from build123d import *

# Parameters (mm, degrees)
BOSS_EXTRUDE4_DEPTH = 50
SKETCH7_R           = 1.75
CUT_EXTRUDE1_DEPTH  = 59.719147195
SKETCH8_R           = 0.75
SKETCH8_W           = 11.8
SKETCH8_H           = 22.5
BOSS_EXTRUDE5_DEPTH = 6
SKETCH9_R           = 4.05
BOSS_EXTRUDE6_DEPTH = 8
FILLET1_R           = 3


with BuildPart() as part:
    # Sketch6 → Boss-Extrude4 (new body)
    with BuildSketch(Plane.XZ):
        with BuildLine():
            Line((-1, 25.784833184), (-1, 12.785954208))
            ThreePointArc((-1, 12.785954208), (-12.825, 0), (-1, -12.785954208))
            Line((-1, -12.785954208), (-1, -25.784833184))
            Line((-1, -25.784833184), (-6, -25.784833184))
            Line((-6, -25.784833184), (-6, -16.784833184))
            ThreePointArc((-6, -16.784833184), (-17.825, 0), (-6, 16.784833184))
            Line((-6, 16.784833184), (-6, 25.784833184))
            Line((-6, 25.784833184), (-1, 25.784833184))
        make_face()
    extrude(amount=BOSS_EXTRUDE4_DEPTH)

    # Sketch7 → Cut-Extrude1 (cut, through all)
    with BuildSketch(Plane(origin=(-1, 0, 0), x_dir=(0, 0, -1), z_dir=(1, 0, 0))):
        with Locations((-19.285393696, -10)):
            Circle(SKETCH7_R)
        with Locations((-19.285393696, -40)):
            Circle(SKETCH7_R)
        with Locations((19.285393696, -40)):
            Circle(SKETCH7_R)
        with Locations((19.285393696, -10)):
            Circle(SKETCH7_R)
    extrude(amount=-CUT_EXTRUDE1_DEPTH, mode=Mode.SUBTRACT)

    # Sketch8 → Boss-Extrude5 (add)
    with BuildSketch(Plane(origin=(0, 0, 0), x_dir=(1, 0, 0), z_dir=(0, 1, 0))):
        with BuildLine():
            Line((-33.34361413, -16.25), (-22.318992281, -16.25))
            ThreePointArc((-22.318992281, -16.25), (-21.069616181, -16.522536094), (-20.047240136, -17.290627093))
            ThreePointArc((-20.047240136, -17.290627093), (26.473715688, 0), (-20.047240136, 17.290627093))
            ThreePointArc((-20.047240136, 17.290627093), (-21.069616181, 16.522536094), (-22.318992281, 16.25))
            Line((-22.318992281, 16.25), (-33.34361413, 16.25))
            ThreePointArc((-33.34361413, 16.25), (-35.464934474, 15.371320344), (-36.34361413, 13.25))
            Line((-36.34361413, 13.25), (-36.34361413, -13.25))
            ThreePointArc((-36.34361413, -13.25), (-35.464934474, -15.371320344), (-33.34361413, -16.25))
        make_face()
        with Locations(Location((-25.44361413, 13.65, 0), (0, 0, 270))):
            Circle(SKETCH8_R, mode=Mode.SUBTRACT)
        with Locations(Location((-25.44361413, -13.65, 0), (0, 0, 270))):
            Circle(SKETCH8_R, mode=Mode.SUBTRACT)
        with Locations((-25.44361413, 0)):
            Rectangle(SKETCH8_W, SKETCH8_H, mode=Mode.SUBTRACT)
    extrude(amount=BOSS_EXTRUDE5_DEPTH)

    # Sketch9 → Boss-Extrude6 (add)
    with BuildSketch(Plane(origin=(0, 6, 0), x_dir=(1, 0, 0), z_dir=(0, 1, 0))):
        with Locations(Location((0, 0, 0), (0, 0, 270))):
            Circle(SKETCH9_R)
    extrude(amount=BOSS_EXTRUDE6_DEPTH)

    # Fillet1
    fillet1_edges = [part.edges().sort_by_distance(p)[0] for p in [
        (0, 6, -4.05),
    ]]
    fillet(fillet1_edges, radius=FILLET1_R)


solid = part.part
Can you work these out from the model? Positions are in its coordinate system, mm. A direction names the side the tool comes from. Give positions to 0.01 mm unless a question says otherwise; leave off trailing zeros. Write each loop counter-clockwise with the first axis right and the second up, starting at its lowest first coordinate (ties: lowest second). Pieces come first, ordered by that corner, then holes. Notation, with made-up numbers: M 19.25,-24 L 60.25,-24 A32 ccw 60.25,2 Z; hole C 24,-32 d10. An arc over 180 degrees is marked long. Answer in a Markdown table with one row per item. Add a question column.
Item 1: On a 3-axis mill with a long thin cutter (end or side, diameter ignored), from which of +Z, -Z, +X, -X, +Y, -Y can I reach the whole of each face in a straight line? I mean faces 1 (the flat face through (-6, -25, -21)), 2 (the flat face through (-6, -25, 21)), 3 (the flat face through (-4, -25, 25.785)), 4 (the flat face through (-19.544, 3, 0)), 5 (the flat face through (-28, 3, -16.25)). Say none if no direction works.
Item 2: We'd pull the mould along Y, two halves only. Please class faces 6 (the cylindrical face through (-35.441, 2.958, -15.395)), 7 (the cylindrical face through (-3.465, -9.474, -20.955)), 8 (the cylindrical face through (-3.5, -41.7, 19.7)), 9 (the flat face through (0, 14, 0)): released by +Y, released by -Y, zero draft, split by the parting line, or undercut.
Item 3: For pin 1 Ø12 at (x, z) = (11.5, 11) entering from -Y; pin 2 Ø3 at (x, y) = (-26, 2) entering from -Z; pin 3 Ø2.5 at (x, y) = (-4.5, -23.5) entering from +Z; pin 4 Ø3 at (y, z) = (-10, -19.29) entering from +X, each with a flat end and sliding along its axis, tell me the tip position at first contact or that it passes through.
Item 4: Imagine slicing it at B-B, the plane y = -4. Write out the boundary of the cut face in (x, z) (3 decimals).
Item 5: Imagine slicing it at D-D, the plane x = 0. Write out the boundary of the cut face in (y, z), plus the area to 3 significant figures.
Item 6: Imagine slicing it at A-A, the plane x = -27.5. Write out the boundary of the cut face in (y, z).
Item 7: Imagine slicing it at C-C, the plane z = 0. Write out the boundary of the cut face in (x, y) (3 decimals), plus the area to 3 significant figures.
Item 8: Please list where these lines run through material, in increasing order: L1, parallel to Z at x = -9, y = -16; L2, parallel to Y at x = -17, z = -16.5; L3, parallel to Y at x = -15, z = -2.5.
Evaluation:
| question | item | result |
|---|---|---|
| 1 | face 1 | -Z, -X, -Y |
| 1 | face 2 | +Z, -X, -Y |
| 1 | face 3 | +Z, +X, -X, -Y |
| 1 | face 4 | +Y, -Y |
| 1 | face 5 | -Z, -X, +Y, -Y |
| 2 | face 6 | zero draft |
| 2 | face 7 | undercut |
| 2 | face 8 | undercut |
| 2 | face 9 | released by +Y |
| 3 | pin 1 | stops at y = 0 |
| 3 | pin 2 | stops at z = -16.25 |
| 3 | pin 3 | stops at z = 25.78 |
| 3 | pin 4 | passes through |
| 4 | outline | M -6,-25.785 L -1,-25.785 L -1,-12.786 A12.825 cw -1,12.786 L -1,25.785 L -6,25.785 L -6,16.785 A17.825 ccw -6,-16.785 Z |
| 5 | outline | M 0,-26.47 L 6,-26.47 L 6,-7.05 A3 cw 9,-4.05 L 14,-4.05 L 14,4.05 L 9,4.05 A3 cw 6,7.05 L 6,26.47 L 0,26.47 Z |
| 5 | area | 386 mm² |
| 6 | outline | M 0,-16.25 L 6,-16.25 L 6,-11.25 L 0,-11.25 Z; M 0,11.25 L 6,11.25 L 6,16.25 L 0,16.25 Z |
| 7 | outline | M -36.344,0 L -31.344,0 L -31.344,6 L -36.344,6 Z; M -19.544,0 L -17.825,0 L -17.825,-50 L -12.825,-50 L -12.825,0 L 26.474,0 L 26.474,6 L 7.05,6 A3 cw 4.05,9 L 4.05,14 L -4.05,14 L -4.05,9 A3 cw -7.05,6 L -19.544,6 Z |
| 7 | area | 625 mm² |
| 8 | L1 | z = -15.39 to -9.14, 9.14 to 15.39 |
| 8 | L2 | y = 0 to 6 |
| 8 | L3 | y = -50 to 6 |
